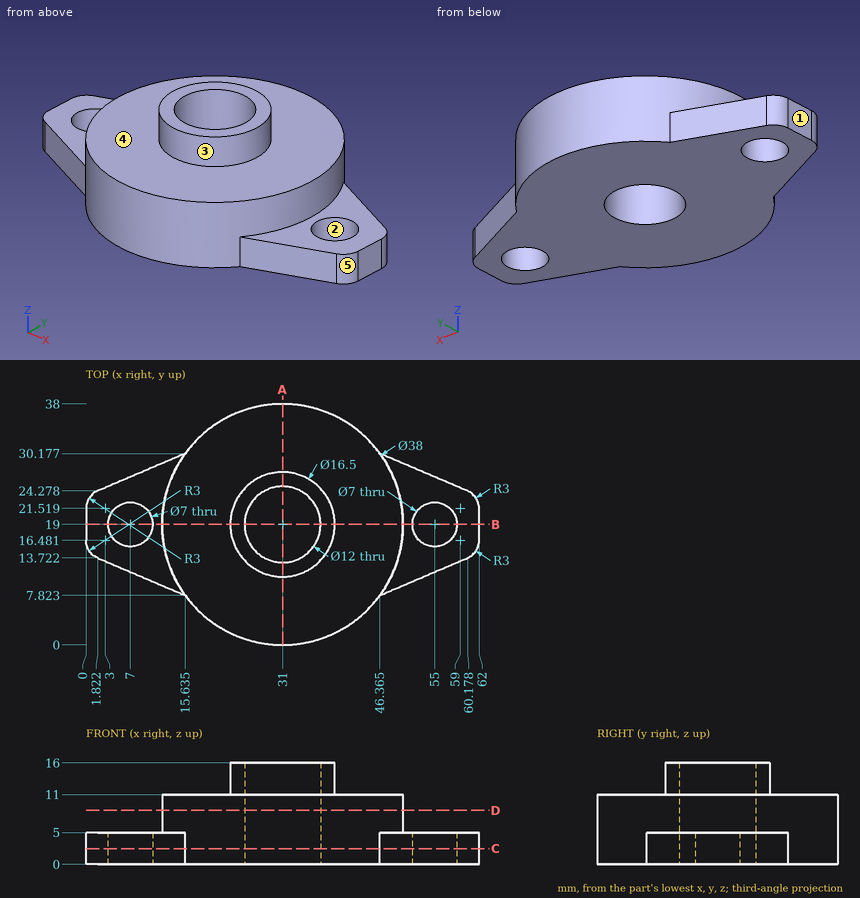
Geometry check sheet. Reference: drawing and pictorial views, mm from the part's lowest x, y, z. A direction names the side the tool comes from. Coordinates: 2 decimals unless noted, no trailing zeros. Loops run counter-clockwise (first coordinate to the right, second up) from the corner with the lowest first, then second, coordinate; pieces in that order, holes last. Notation, with made-up numbers: M 14,-29 L 28,-29 A28 cw 28,4 Z; hole C -35.75,-7.5 d4. An arc over 180 degrees is marked long. One line per item, written item: value.
1. Set-up check for the marked faces 4 and 5: record each of +Z, -Z, +X, -X, +Y, -Y from which the full face is reachable in a straight line by a thin tool's end or side.
Answers follow:
face 4: +Z
face 5: +Z, -Z, +X, -Y
2. Section check B-B on y = 19. Record the cut outline in (x, z).
Answers follow:
outline: M 0,0 L 3.5,0 L 3.5,5 L 0,5 Z; M 10.5,0 L 25,0 L 25,16 L 22.75,16 L 22.75,11 L 12,11 L 12,5 L 10.5,5 Z; M 37,0 L 51.5,0 L 51.5,5 L 50,5 L 50,11 L 39.25,11 L 39.25,16 L 37,16 Z; M 58.5,0 L 62,0 L 62,5 L 58.5,5 Z
3. Material ranges on line 1 along Y through (x, z) = (31, 12.25); line 2 along Y through (x, z) = (31, 6.5); line 3 along Z through (x, y) = (15, 24), recorded low to high. Write a range as from..to.
Answers follow:
line 1: 10.75..13, 25..27.25
line 2: 0..13, 25..38
line 3: 0..11
4. Gauge pin test, flat ends, axial feed: P1, Ø6, axis at x = 30.5, z = 7.5, coming from the -Y side; P2, Ø1.5, axis at x = 17, z = 10, coming from the -Y side; P3, Ø8, axis at x = 46, z = 10, coming from the +Y side. Record the tip position at first contact, or that the pin passes through.
Answers follow:
P1: y = 0
P2: y = 5.38
P3: y = 34.49
5. Section check D-D on z = 8.5. Record the cut outline in (x, y).
Answers follow:
outline: C 31,19 d38; hole C 31,19 d12
6. Section check C-C on z = 2.5. Record the cut outline in (x, y) (1 decimal).
Answers follow:
outline: M 0,16.5 A3 ccw 1.8,13.7 L 15.6,7.8 A19 ccw 46.4,7.8 L 60.2,13.7 A3 ccw 62,16.5 L 62,21.5 A3 ccw 60.2,24.3 L 46.4,30.2 A19 ccw 15.6,30.2 L 1.8,24.3 A3 ccw 0,21.5 Z; hole C 7,19 d7; hole C 31,19 d12; hole C 55,19 d7
7. Section check A-A on x = 31. Record the cut outline in (y, z).
Answers follow:
outline: M 0,0 L 13,0 L 13,16 L 10.75,16 L 10.75,11 L 0,11 Z; M 25,0 L 38,0 L 38,11 L 27.25,11 L 27.25,16 L 25,16 Z
8. Mould release check, pull along X, two halves, no side actions. Record for the marked faces 1, 2 and 3: pulls with the +X half, pulls with the -X half, needs draft (parallel to the pull), parting line crosses it, or undercut.
Answers follow:
face 1: pulls with the -X half
face 2: undercut
face 3: parting line crosses it
